```python
from build123d import *

# Parameters (mm, degrees)
SKETCH_W        = 46
SKETCH_H        = 13.6
SKETCH_R        = 1.7
PAD_DEPTH       = 4
PAD001_DEPTH    = 4
SKETCH002_W     = 4.3
SKETCH002_H     = 1.7
POCKET_DEPTH    = 10
SKETCH003_W     = 16.5
SKETCH003_H     = 7.2
POCKET001_DEPTH = 4
SKETCH004_W     = 3
SKETCH004_H     = 1.5
POCKET002_DEPTH = 110.862709
FILLET_R        = 2
FILLET001_R     = 2
CHAMFER_SIZE    = 1.5
CHAMFER001_SIZE = 1.5


with BuildPart() as part:
    # Sketch → Pad (new body)
    with BuildSketch(Plane.XY):
        Rectangle(SKETCH_W, SKETCH_H)
        with Locations((-17.5, 0)):
            Circle(SKETCH_R, mode=Mode.SUBTRACT)
        with Locations((17.5, 0)):
            Circle(SKETCH_R, mode=Mode.SUBTRACT)
    extrude(amount=-PAD_DEPTH)

    # Sketch001 → Pad001 (new body)
    with BuildSketch(Plane.XY):
        with BuildLine():
            ThreePointArc((-4.75, 6.8), (-11.55, 0), (-4.75, -6.8))
            Line((-4.75, -6.8), (4.75, -6.8))
            ThreePointArc((4.75, -6.8), (11.55, 0), (4.75, 6.8))
            Line((-4.75, 6.8), (4.75, 6.8))
        make_face()
    extrude(amount=PAD001_DEPTH)

    # Sketch002 → Pocket (cut)
    with BuildSketch(Plane.XZ.offset(6.8)):
        Polygon((-7.066496, 2.040643), (-2.814518, 1.399799), (-3.067875, -0.281215), (-7.319853, 0.359629), align=None)
        with Locations((0, 0.5)):
            Rectangle(SKETCH002_W, SKETCH002_H)
        Polygon((2.814518, 1.399799), (7.066496, 2.040644), (7.319853, 0.359629), (3.067875, -0.281216), align=None)
    extrude(amount=-POCKET_DEPTH, mode=Mode.SUBTRACT)

    # Sketch003 → Pocket001 (cut)
    with BuildSketch(Plane.XZ.offset(6.8)):
        with Locations((0, -1.1)):
            Rectangle(SKETCH003_W, SKETCH003_H)
    extrude(amount=-POCKET001_DEPTH, mode=Mode.SUBTRACT)

    # Sketch004 → Pocket002 (cut, through all)
    with BuildSketch(Plane.XZ.offset(6.8)):
        with Locations((-13, -0.75)):
            Rectangle(SKETCH004_W, SKETCH004_H)
    pocket002 = extrude(amount=-POCKET002_DEPTH, mode=Mode.SUBTRACT)

    # Mirrored: Pocket002 across Sketch004 V_Axis
    add(pocket002.mirror(Plane(origin=(0, -6.8, 0), x_dir=(0, -1, 0), z_dir=(1, 0, 0))), mode=Mode.SUBTRACT)

    # Fillet
    fillet_edges = [part.edges().sort_by_distance(p)[0] for p in [
        (-23, 0, -4),
    ]]
    fillet(fillet_edges, radius=FILLET_R)

    # Fillet001
    fillet001_edges = [part.edges().sort_by_distance(p)[0] for p in [
        (23, 0, -4),
    ]]
    fillet(fillet001_edges, radius=FILLET001_R)

    # Chamfer
    chamfer_edges = [part.edges().sort_by_distance(p)[0] for p in [
        (-19.2, 0, -4),
    ]]
    chamfer(chamfer_edges, length=CHAMFER_SIZE)

    # Chamfer001
    chamfer001_edges = [part.edges().sort_by_distance(p)[0] for p in [
        (15.8, 0, -4),
    ]]
    chamfer(chamfer001_edges, length=CHAMFER001_SIZE)


solid = part.part
```
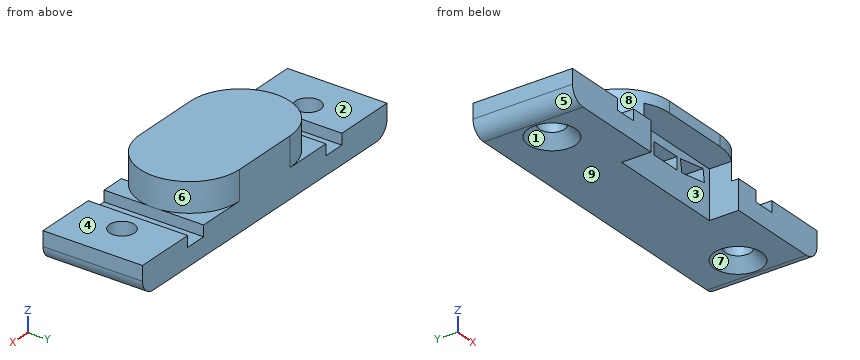
Design review of the part built by this model. Coordinates are the model's own, in mm. Face numbers are marked on the shaded views. A direction names the side the tool comes from. Give positions to 0.01 mm unless a question says otherwise; leave off trailing zeros. Write each loop counter-clockwise with the first axis right and the second up, starting at its lowest first coordinate (ties: lowest second). Pieces come first, ordered by that corner, then holes. Notation, with made-up numbers: (42.5, 13) - (59.5, 13) arc R17 ccw to (59.5, 29) - close; hole circle Ø8 at (-1, -31.5). An arc over 180 degrees is marked (long way). Return JSON: item names as keys, results as strings. Group by question number.
(1) We need section B-B, the plane x = 0.5. Give the boundary of the cut face in (y, z).
(2) Machinability: for the marked faces 1, 2, 3, 4 and 5, which of the approach directions +Z, -Z, +X, -X, +Y, -Y give a long, thin tool a straight path to every point of the face, cutting with its end or side? Answer none if there is none.
(3) To check wall thickness, follow probe 1 along X at (y, z) = (-5.75, -0.5); probe 2 along Z at (x, y) = (1, -1.75); probe 3 along X at (y, z) = (-5, -2). State the ranges of each line that lie inside material, in increasing order.
(4) We need section C-C, the plane y = 3.75. Give the boundary of the cut face in (x, z).
(5) We need section D-D, the plane z = -3.25. Give the boundary of the cut face in (x, y).
(6) Mouldability with a two-part tool opening along X and no side actions: class the marked faces 6, 7, 8 and 9 as +X half, -X half, draft (parallel to the pull), parting line (faces both ways), or undercut.
(7) We need section A-A, the plane x = -17.5. Give the boundary of the cut face in (y, z), then the cut area to 4 significant figures.
(8) Insertion check: pin 1 (4 mm diameter, centred on x = -17.5, y = 0, fed in from -Z); pin 2 (0.9 mm diameter, centred on x = -12.5, y = 3.5, fed in from +Z); pin 3 (7 mm diameter, centred on x = 16.5, y = -2, fed in from +Z). Each pin has a flat end and moves straight along its axis. Give the tip position at first contact, or say it passes through.
Reported:
{
 "1": {"outline": "(-6.8, 2.5) - (-2.8, 2.5) - (-2.8, 1.35) - (3.2, 1.35) - (3.2, -0.35) - (-2.8, -0.35) - (-2.8, -4) - (6.8, -4) - (6.8, 4) - (-6.8, 4) - close"},
 "2": {"face 1": "-Z", "face 2": "+Z, -X, +Y, -Y", "face 3": "-Z, -Y", "face 4": "+Z, +X, +Y, -Y", "face 5": "-Z, -X, +Y, -Y"},
 "3": {"probe 1": "x = -23 to -14.5, -11.5 to -8.25, 8.25 to 11.5, 14.5 to 23", "probe 2": "z = -4 to -0.35, 1.35 to 4", "probe 3": "x = -23 to -8.25, 8.25 to 23"},
 "4": {"outline": "(-23, -2) arc R2 ccw to (-21, -4) - (21, -4) arc R2 ccw to (23, -2) - (23, 0) - (14.5, 0) - (14.5, -1.5) - (11.5, -1.5) - (11.5, 0) - (10.42, 0) - (10.42, 4) - (-10.42, 4) - (-10.42, 0) - (-11.5, 0) - (-11.5, -1.5) - (-14.5, -1.5) - (-14.5, 0) - (-23, 0) - close"},
 "5": {"outline": "(-22.56, -6.8) - (-8.25, -6.8) - (-8.25, -2.8) - (8.25, -2.8) - (8.25, -6.8) - (22.56, -6.8) - (22.56, 6.8) - (-22.56, 6.8) - close; hole circle Ø4.9 at (-17.5, 0); hole circle Ø4.9 at (17.5, 0)"},
 "6": {"face 6": "+X half", "face 7": "undercut", "face 8": "-X half", "face 9": "draft"},
 "7": {"outline": "(-6.8, -4) - (-3.2, -4) - (-1.7, -2.5) - (-1.7, 0) - (-6.8, 0) - close; (1.7, -2.5) - (3.2, -4) - (6.8, -4) - (6.8, 0) - (1.7, 0) - close", "area": "38.55 mm2"},
 "8": {"pin 1": "stops at z = -2.8", "pin 2": "stops at z = -1.5", "pin 3": "stops at z = 0"}
}
